```python
from build123d import *

# Parameters (mm, degrees)
F0_R          = 12.5
F0_R_2        = 6
F1_DEPTH      = 25
F3_R          = 12
F3_R_2        = 6
F4_DEPTH      = 12.5
F4_DEPTH_BACK = 12.5
F5_R          = 7.5
F7_R          = 6
F8_DEPTH      = 12.5010001
F8_DEPTH_BACK = 25.0010001


with BuildPart() as f1:
    # F0 (on Top) → F1 (new body)
    with BuildSketch(Plane.XY):
        Circle(F0_R)
        Circle(F0_R_2, mode=Mode.SUBTRACT)
    extrude(amount=F1_DEPTH)



with BuildPart() as f4:
    # F3 (on Top) → F4 (new body, two sides)
    with BuildSketch(Plane.XY) as f4_sk:
        with Locations((150, 0)):
            Circle(F3_R)
        with Locations((150, 0)):
            Circle(F3_R_2, mode=Mode.SUBTRACT)
    extrude(amount=F4_DEPTH)
    extrude(f4_sk.sketch, amount=-F4_DEPTH_BACK)


with BuildPart() as f1_1:
    add(f1.part)

    add(f4.part)  # F6 merges F4
    # F6: sweep along a path in F2
    with BuildLine(Plane.XZ) as f6_path:
        Line((0, 12), (25, 12))
        ThreePointArc((25, 12), (32.1487132371, 11.5726103092), (39.1955835962, 10.2965299685))
        ThreePointArc((39.1955835962, 10.2965299685), (81.789999989, 2.5833332421), (125, 0))
        Line((125, 0), (150, 0))
    # F5 (on Right) → F6 (sweep)
    with BuildSketch(Plane.YZ):
        with Locations((0, 12)):
            Circle(F5_R)
    sweep(path=f6_path.line)

    # F7 (on Top) → F8 (cut, two sides)
    with BuildSketch(Plane.XY) as f8_sk:
        Circle(F7_R)
        with Locations((150, 0)):
            Circle(F7_R)
    extrude(amount=-F8_DEPTH, mode=Mode.SUBTRACT)
    extrude(f8_sk.sketch, amount=F8_DEPTH_BACK, mode=Mode.SUBTRACT)


solid = f1_1.part
```
Work out the finished part from the listing and answer in its coordinate system (mm). A direction names the side the tool comes from. Round coordinates to 2 decimals unless told otherwise and drop trailing zeros. Write each loop counter-clockwise with the first axis right and the second up, starting at its lowest first coordinate (ties: lowest second). Pieces come first, ordered by that corner, then holes. Notation, with made-up numbers: (11.25, 79.25) -> (36.25, 79.25) arc R15 cw to (36.25, 97.25) -> close; hole circle Ø10 at (-40, -11.75). An arc over 180 degrees is marked (long way). Write each question's results on one line, items separated by ' | '.
1) Flat-ended cylindrical pins translate along their axes: pin 1 (1 mm diameter, centred on x = 62.5, z = -0.5, fed in from +Y); pin 2 (12 mm diameter, centred on x = 128, y = 10, fed in from +Z); pin 3 (6 mm diameter, centred on x = 16, y = 0.5, fed in from +Z). Find the tip coordinate at first contact, or state that the pin passes through.
Findings:
pin 1: stops at y = 5.27 | pin 2: stops at z = 6.34 | pin 3: stops at z = 19.5
2) Which of the six approach directions +Z, -Z, +X, -X, +Y, -Y give full straight-line access (tool end or side, diameter ignored) to faces 1 (the flat face through (152, 6, 12.5)), 2 (the flat face through (-3, -5.4, 0)), 3 (the cylindrical face through (132.926, 7.154, 2.253))?
Findings:
face 1: +Z, +X, +Y, -Y | face 2: -Z, -X, +Y, -Y | face 3: none
3) The part is cut by section C-C (z = -9). Write down the section's boundary in (x, y).
Findings:
outline: circle Ø24 at (150, 0); hole circle Ø12 at (150, 0)
4) The part is cut by section D-D (x = 150). Write down the section's boundary in (y, z).
Findings:
outline: (-12, -12.5) -> (-6, -12.5) -> (-6, 12.5) -> (-12, 12.5) -> close; (6, -12.5) -> (12, -12.5) -> (12, 12.5) -> (6, 12.5) -> close
5) For a pull along X with two mould halves and no side action, classify faces 4 (the cylindrical face through (145.24, -3.65, -0.18)), 5 (the cylindrical face through (-12.488, 0.55, 12.325)), 6 (the flat face through (-3, -5.4, 25)) as +X half, -X half, draft (parallel to the pull), parting line (faces both ways), or undercut.
Findings:
face 4: undercut | face 5: undercut | face 6: draft
6) Consider line 1 along Y through (x, z) = (150, -7.5); line 2 along Y through (x, z) = (0, 10); line 3 along Z through (x, y) = (155.5, -6.25). Determine where each line is inside the solid, lowest interval first. Write a range as [from, to].
Findings:
line 1: y = [-12, -6], [6, 12] | line 2: y = [-12.5, -6], [6, 12.5] | line 3: z = [-12.5, 12.5]
7) The part is cut by section A-A (x = 0). Write down the section's boundary in (y, z).
Findings:
outline: (-12.5, 0) -> (-6, 0) -> (-6, 25) -> (-12.5, 25) -> close; (6, 0) -> (12.5, 0) -> (12.5, 25) -> (6, 25) -> close
8) The part is cut by section B-B (y = 0). Write down the section's boundary in (x, z).
Findings:
outline: (-12.5, 0) -> (-6, 0) -> (-6, 25) -> (-12.5, 25) -> close; (6, 0) -> (12.5, 0) -> (12.5, 4.5) -> (25, 4.5) arc R52.5 cw to (37.42, 3.01) arc R370.17 ccw to (125, -7.5) -> (138, -7.5) -> (138, -12.5) -> (144, -12.5) -> (144, 12.5) -> (138, 12.5) -> (138, 7.5) -> (125, 7.5) arc R355.17 cw to (40.97, 17.58) arc R67.5 ccw to (25, 19.5) -> (12.5, 19.5) -> (12.5, 25) -> (6, 25) -> close; (156, -12.5) -> (162, -12.5) -> (162, 12.5) -> (156, 12.5) -> close
